from build123d import *

# Parameters (mm, degrees)
SKETCH1_R            = 4.445
BOSS_EXTRUDE1_DEPTH  = 114.3
BOSS_EXTRUDE3_DEPTH  = 38.1
SKETCH13_W           = 47.954543922
SKETCH13_H           = 15.24
BOSS_EXTRUDE4_DEPTH  = 50.8
BOSS_EXTRUDE5_DEPTH  = 7.62
BOSS_EXTRUDE6_DEPTH  = 8.382
BOSS_EXTRUDE7_DEPTH  = 76.2
BOSS_EXTRUDE8_DEPTH  = 7.62
BOSS_EXTRUDE9_DEPTH  = 8.382
BOSS_EXTRUDE10_DEPTH = 73.66
BOSS_EXTRUDE11_DEPTH = 73.406
SKETCH23_W           = 19.757692601
SKETCH23_H           = 17.78
CUT_EXTRUDE11_DEPTH  = 20.32
SKETCH24_R           = 10.16
CUT_EXTRUDE12_DEPTH  = 50.8
SKETCH25_W           = 23.730892102
SKETCH25_H           = 8.382
CUT_EXTRUDE14_DEPTH  = 12.7
SKETCH26_W           = 33.02
SKETCH26_H           = 76.2
BOSS_EXTRUDE13_DEPTH = 57.15
SKETCH34_R           = 1.524
CUT_EXTRUDE18_DEPTH  = 5.08
SKETCH35_R           = 1.524
CUT_EXTRUDE19_DEPTH  = 5.08
SKETCH36_R           = 1.524
CUT_EXTRUDE20_DEPTH  = 5.08
SKETCH37_W           = 21.59
SKETCH37_H           = 34.29
CUT_EXTRUDE21_DEPTH  = 50.8
SKETCH38_R           = 1.524
CUT_EXTRUDE22_DEPTH  = 10.16
CUT_EXTRUDE23_DEPTH  = 5.08


with BuildPart() as part:
    # Sketch1 → Boss-Extrude1 (new body)
    with BuildSketch(Plane(origin=(0, 0, 0), x_dir=(1, 0, 0), z_dir=(0, 1, 0))):
        with BuildLine():
            Line((0, 7.62), (127, 7.62))
            ThreePointArc((127, 7.62), (134.62, 0), (127, -7.62))
            Line((127, -7.62), (76.2, -7.62))
            Line((76.2, -7.62), (76.2, -64.77))
            Line((76.2, -64.77), (69.85, -64.77))
            Line((69.85, -64.77), (69.85, -7.62))
            Line((69.85, -7.62), (0, -7.62))
            ThreePointArc((0, -7.62), (-7.62, 0), (0, 7.62))
        make_face()
        with Locations(Location((0, 0, 0), (0, 0, 270))):
            Circle(SKETCH1_R, mode=Mode.SUBTRACT)
        with Locations(Location((127, 0, 0), (0, 0, 270))):
            Circle(SKETCH1_R, mode=Mode.SUBTRACT)
    extrude(amount=BOSS_EXTRUDE1_DEPTH)

    # Sketch12 → Boss-Extrude3 (add)
    with BuildSketch(Plane(origin=(0, 114.3, 0), x_dir=(1, 0, 0), z_dir=(0, 1, 0))):
        Polygon((69.85, -7.62), (69.85, -64.77), (21.895456078, -7.62), align=None)
    extrude(amount=-BOSS_EXTRUDE3_DEPTH)

    # Sketch13 → Boss-Extrude4 (add)
    with BuildSketch(Plane(origin=(0, 114.3, 0), x_dir=(1, 0, 0), z_dir=(0, 1, 0))):
        with Locations((45.872728039, 0)):
            Rectangle(SKETCH13_W, SKETCH13_H)
        Polygon((69.85, -7.62), (69.85, -64.77), (21.895456078, -7.62), align=None)
    extrude(amount=BOSS_EXTRUDE4_DEPTH)

    # Sketch14 → Boss-Extrude5 (add)
    with BuildSketch(Plane.XZ.offset(-76.2)):
        Polygon((21.895456078, 7.62), (69.85, 64.77), (53.271327425, 64.77), (12.166691651, 15.783402643), (5.316783504, 7.62), align=None)
    extrude(amount=-BOSS_EXTRUDE5_DEPTH)

    # Sketch15 → Boss-Extrude6 (add)
    with BuildSketch(Plane(origin=(0, 165.1, 0), x_dir=(1, 0, 0), z_dir=(0, 1, 0))):
        Polygon((69.85, -64.77), (53.271327425, -64.77), (5.316783504, -7.62), (5.316783504, 7.62), (21.895456078, 7.62), (21.895456078, -7.62), align=None)
    extrude(amount=-BOSS_EXTRUDE6_DEPTH)

    # Sketch17 → Boss-Extrude7 (add)
    with BuildSketch(Plane.XZ.offset(-156.718)):
        Polygon((12.166691651, 15.783402643), (5.316783504, 7.62), (5.316783504, -7.62), (21.895456078, -7.62), (21.895456078, 7.62), (25.160817135, 11.511505771), (15.432052708, 19.674908414), align=None)
    extrude(amount=BOSS_EXTRUDE7_DEPTH)

    # Sketch18 → Boss-Extrude8 (add)
    with BuildSketch(Plane.XZ.offset(-76.2)):
        Polygon((5.316783504, 7.62), (5.316783504, 27.377692601), (36.692654851, 64.77), (53.271327425, 64.77), align=None)
    extrude(amount=-BOSS_EXTRUDE8_DEPTH)

    # Sketch19 → Boss-Extrude9 (add)
    with BuildSketch(Plane(origin=(0, 165.1, 0), x_dir=(1, 0, 0), z_dir=(0, 1, 0))):
        Polygon((5.316783504, -7.62), (5.316783504, -27.377692601), (36.692654851, -64.77), (53.271327425, -64.77), align=None)
    extrude(amount=-BOSS_EXTRUDE9_DEPTH)

    # Sketch20 → Boss-Extrude10 (add)
    with BuildSketch(Plane.XZ.offset(-156.718)):
        Polygon((15.432052708, 19.674908414), (5.316783504, 27.377692601), (5.316783504, 7.62), align=None)
    extrude(amount=BOSS_EXTRUDE10_DEPTH)

    # Sketch22 → Boss-Extrude11 (add)
    with BuildSketch(Plane.XZ.offset(-156.718)):
        Polygon((69.85, 64.77), (58.094700194, 50.760579224), (41.398922654, 64.77), align=None)
    extrude(amount=BOSS_EXTRUDE11_DEPTH)

    # Sketch23 → Cut-Extrude11 (cut)
    with BuildSketch(Plane.ZY.offset(-5.316783504)):
        with Locations((17.498846301, 105.41)):
            Rectangle(SKETCH23_W, SKETCH23_H)
    extrude(amount=-CUT_EXTRUDE11_DEPTH, mode=Mode.SUBTRACT)

    # Sketch24 → Cut-Extrude12 (cut)
    with BuildSketch(Plane(origin=(0, 165.1, 0), x_dir=(1, 0, 0), z_dir=(0, 1, 0))):
        Circle(SKETCH24_R)
    extrude(amount=-CUT_EXTRUDE12_DEPTH, mode=Mode.SUBTRACT)

    # Sketch25 → Cut-Extrude14 (cut)
    with BuildSketch(Plane.XY.offset(64.77)):
        Polygon((41.398922654, 114.3), (69.85, 114.3), (69.85, 165.1), (36.692654851, 165.1), (36.692654851, 156.718), (41.398922654, 156.718), align=None)
        with Locations((24.8272088, 160.909)):
            Rectangle(SKETCH25_W, SKETCH25_H)
    extrude(amount=-CUT_EXTRUDE14_DEPTH, mode=Mode.SUBTRACT)

    # Sketch26 → Boss-Extrude13 (add)
    with BuildSketch(Plane.XY.offset(7.62)):
        with Locations((53.34, 38.1)):
            Rectangle(SKETCH26_W, SKETCH26_H)
    extrude(amount=BOSS_EXTRUDE13_DEPTH)

    # Sketch34 → Cut-Extrude18 (cut)
    with BuildSketch(Plane(origin=(0, 0, -7.62), x_dir=(-1, 0, 0), z_dir=(0, 0, -1))):
        with Locations((-109.22, 95.25)):
            Circle(SKETCH34_R)
        with Locations((-95.25, 95.25)):
            Circle(SKETCH34_R)
        with Locations((-95.25, 63.5)):
            Circle(SKETCH34_R)
        with Locations((-109.22, 63.5)):
            Circle(SKETCH34_R)
        with Locations((-109.22, 44.45)):
            Circle(SKETCH34_R)
        with Locations((-95.25, 44.45)):
            Circle(SKETCH34_R)
        with Locations((-109.22, 12.7)):
            Circle(SKETCH34_R)
        with Locations((-95.25, 12.7)):
            Circle(SKETCH34_R)
    extrude(amount=-CUT_EXTRUDE18_DEPTH, mode=Mode.SUBTRACT)

    # Sketch35 → Cut-Extrude19 (cut)
    with BuildSketch(Plane.XY.offset(7.62)):
        with Locations((102.87, 92.71)):
            Circle(SKETCH35_R)
        with Locations((116.84, 92.71)):
            Circle(SKETCH35_R)
        with Locations((102.87, 63.5)):
            Circle(SKETCH35_R)
        with Locations((116.84, 63.5)):
            Circle(SKETCH35_R)
        with Locations((101.6, 19.05)):
            Circle(SKETCH35_R)
        with Locations((116.84, 19.05)):
            Circle(SKETCH35_R)
    extrude(amount=-CUT_EXTRUDE19_DEPTH, mode=Mode.SUBTRACT)

    # Sketch36 → Cut-Extrude20 (cut)
    with BuildSketch(Plane(origin=(76.2, 0, 0), x_dir=(0, 0, -1), z_dir=(1, 0, 0))):
        with Locations((-59.69, 6.35)):
            Circle(SKETCH36_R)
        with Locations((-46.99, 6.35)):
            Circle(SKETCH36_R)
        with Locations((-46.99, 31.75)):
            Circle(SKETCH36_R)
        with Locations((-59.69, 31.75)):
            Circle(SKETCH36_R)
    extrude(amount=-CUT_EXTRUDE20_DEPTH, mode=Mode.SUBTRACT)

    # Sketch37 → Cut-Extrude21 (cut)
    with BuildSketch(Plane.XZ):
        with Locations((57.785, 24.765)):
            Rectangle(SKETCH37_W, SKETCH37_H)
    extrude(amount=-CUT_EXTRUDE21_DEPTH, mode=Mode.SUBTRACT)

    # Sketch38 → Cut-Extrude22 (cut)
    with BuildSketch(Plane.XZ):
        with Locations(Location((57.785, 48.26, 0), (0, 0, 270))):
            Circle(SKETCH38_R)
        with Locations(Location((57.785, 2.54, 0), (0, 0, 270))):
            Circle(SKETCH38_R)
    extrude(amount=-CUT_EXTRUDE22_DEPTH, mode=Mode.SUBTRACT)

    # Sketch39 → Cut-Extrude23 (cut)
    with BuildSketch(Plane(origin=(0, 0, -7.62), x_dir=(-1, 0, 0), z_dir=(0, 0, -1))):
        with BuildLine():
            ThreePointArc((-55.88, 102.87), (-57.15, 104.14), (-58.42, 102.87))
            Line((-58.42, 102.87), (-55.88, 102.87))
        make_face()
        with BuildLine():
            Line((-55.88, 102.87), (-58.42, 102.87))
            ThreePointArc((-58.42, 102.87), (-57.15, 101.6), (-55.88, 102.87))
        make_face()
        with BuildLine():
            ThreePointArc((-58.42, 39.37), (-57.15, 38.1), (-55.88, 39.37))
            Line((-55.88, 39.37), (-58.42, 39.37))
        make_face()
        with BuildLine():
            Line((-58.42, 39.37), (-55.88, 39.37))
            ThreePointArc((-55.88, 39.37), (-57.15, 40.64), (-58.42, 39.37))
        make_face()
        with BuildLine():
            ThreePointArc((-74.93, 71.12), (-75.301974388, 72.018025612), (-76.2, 72.39))
            Line((-76.2, 72.39), (-76.2, 69.85))
            ThreePointArc((-76.2, 69.85), (-75.301974388, 70.221974388), (-74.93, 71.12))
        make_face()
        with BuildLine():
            Line((-76.2, 69.85), (-76.2, 72.39))
            ThreePointArc((-76.2, 72.39), (-77.47, 71.12), (-76.2, 69.85))
        make_face()
    extrude(amount=-CUT_EXTRUDE23_DEPTH, mode=Mode.SUBTRACT)


solid = part.part
For this review, take the finished solid that the model builds, in its own axes (mm). A direction names the side the tool comes from. Round coordinates to 2 decimals unless told otherwise and drop trailing zeros. Write each loop counter-clockwise with the first axis right and the second up, starting at its lowest first coordinate (ties: lowest second). Pieces come first, ordered by that corner, then holes. Notation, with made-up numbers: M 81,48 L 116,48 A14 cw 116,63 Z; hole C -22.5,37 d6. An arc over 180 degrees is marked long. Write item = value, one per line. Start each with the question number.
(1) The part is to be moulded in two halves that separate along Z. For faces 5 (the face through (5, 114.3, 0)), 6 (the face through (57, 146, 52.07)), 7 (the face through (85, 114.3, 7)), say which applies: +Z half, -Z half, draft (parallel to the pull), parting line (faces both ways), or undercut.
(2) We need section B-B (x = 84). Give the boundary of the cut face in (y, z), then the cut area to 3 significant figures.
(3) We need section D-D (z = 17). Give the boundary of the cut face in (x, y), then the cut area to 3 significant figures.
(4) For faces 1 (the face through (102, 56, 7.62)), 2 (the face through (32, 83.82, 39)), 3 (the face through (58, 25, 7.62)), 4 (the face through (10.45, 135.81, 23.47)), list the 3-axis set-ups (+Z, -Z, +X, -X, +Y, -Y) from which the entire face can be reached by the end or side of a thin tool; tool diameter is ignored.
(5) For line 1 along Y through (x, z) = (95.25, -5.85); line 2 along X through (y, z) = (55, 0) (3 decimals); line 3 along Y through (x, z) = (57.15, -4.55), list the stretches that pass through material, from the lowest coordinate up.
(6) We need section C-C (y = 127). Give the boundary of the cut face in (x, z), then the cut area to 3 significant figures.
(7) We need section A-A (z = 31). Give the boundary of the cut face in (x, y).
(8) Clearance check with flat-ended pins moving along their axes: pin 1 Ø2 at (x, y) = (57.15, 39.37) entering from -Z; pin 2 Ø8 at (x, z) = (0, 0) entering from +Y; pin 3 Ø1.5 at (x, z) = (53, 10.5) entering from -Y; pin 4 Ø0.9 at (x, z) = (58, 3) entering from -Y. State where each tip first meets the part, or that it passes through.
Results found:
q1.face_5 = undercut
q1.face_6 = +Z half
q1.face_7 = draft
q2.outline = M 0,-7.62 L 114.3,-7.62 L 114.3,7.62 L 0,7.62 Z
q2.area = 1,740 mm²
q3.outline = M 5.32,76.2 L 36.83,76.2 L 36.83,0 L 46.99,0 L 46.99,50.8 L 68.58,50.8 L 68.58,0 L 76.2,0 L 76.2,114.3 L 69.85,114.3 L 69.85,165.1 L 5.32,165.1 L 5.32,114.3 L 18.62,114.3 L 18.62,156.72 L 29.77,156.72 L 29.77,83.82 L 18.62,83.82 L 18.62,96.52 L 5.32,96.52 Z
q3.area = 6,830 mm²
q4.face_1 = +Z, +X, +Y, -Y
q4.face_2 = none
q4.face_3 = -Y
q4.face_4 = +Z
q5.line_1 = 0 to 11.18, 14.22 to 42.93, 45.97 to 61.98, 65.02 to 93.73, 96.77 to 114.3
q5.line_2 = -7.62 to -4.445, 4.445 to 122.555, 131.445 to 134.62
q5.line_3 = 0 to 38.1, 40.64 to 101.6, 104.14 to 165.1
q6.outline = M 5.32,8.66 A10.16 cw 6.72,-7.62 L 69.85,-7.62 L 69.85,52.07 L 56.53,52.07 L 58.09,50.76 L 25.16,11.51 L 15.43,19.67 L 5.32,27.38 Z
q6.area = 2,460 mm²
q7.outline = M 8.36,76.2 L 36.83,76.2 L 36.83,0 L 46.99,0 L 46.99,50.8 L 68.58,50.8 L 68.58,0 L 76.2,0 L 76.2,114.3 L 69.85,114.3 L 69.85,165.1 L 8.36,165.1 L 8.36,156.72 L 41.51,156.72 L 41.51,83.82 L 8.36,83.82 Z
q8.pin_1 = -2.54
q8.pin_2 = through
q8.pin_3 = 50.8
q8.pin_4 = 10.16
